Source: CAD feature listing. Evaluate the final solid. Frame: model axes, mm. A direction names the side the tool comes from. Coordinates: 2 decimals unless noted, no trailing zeros. Write each loop counter-clockwise with the first axis right and the second up, starting at its lowest first coordinate (ties: lowest second). Pieces come first, ordered by that corner, then holes. Notation, with made-up numbers: M -38,48.5 L -31,48.5 A26 ccw -31,83.5 Z; hole C 2,52.5 d3. An arc over 180 degrees is marked long. Write item = value, one per line. Start each with the question number.
1. Access query for faces 4 (the face through (4, 84, 3)), 5 (the face through (0, 17, 3)), 6 (the face through (16, 82, 3)). Directions: +Z, -Z, +X, -X, +Y, -Y. A direction counts if a zero-diameter tool reaches every point of the face in a straight line with its end or side. Return the directions, or none.
2. Pull-direction query (Y, two-part tool) for faces 1 (the face through (19.14, 165.1, 3.04)), 2 (the face through (20, 149, 3)), 3 (the face through (3.22, 127.72, 3.04)); classes: pulls with the +Y half, pulls with the -Y half, needs draft (parallel to the pull), parting line crosses it, or undercut.
3. Line query: line 1 along X through (y, z) = (91, 2.1); line 2 along Y through (x, z) = (18.5, 0.3); line 3 along Y through (x, z) = (18.25, 3.75). Output: solid intervals per line, ascending.
4. Section query A-A (z = 3.55). Output: boundary loops of the cut face in (x, y).
5. Section query B-B (y = 95). Output: boundary loops of the cut face in (x, z), then the cut area to 3 significant figures.
Autodesk Inventor part; units mm, degrees
ref_plane "YZ Plane" through (0, 0, 0) normal (1, 0, 0) x (0, 1, 0)
ref_plane "XZ Plane" through (0, 0, 0) normal (0, 1, 0) x (-1, 0, 0)
ref_plane "XY Plane" through (0, 0, 0) normal (0, 0, 1) x (1, 0, 0)
sketch "Skizze1" plane through (0, 0, 0) normal (0, 0, 1) x (1, 0, 0)
  line L0 (0, 0) -> (20, 0)
  line L1 (20, 0) -> (20, 30)
  line L2 (20, 30) -> (0, 30)
  line L3 (0, 30) -> (0, 0)
  line L4 (4, 38) -> (16, 38)
  line L5 (16, 38) -> (16, 128)
  line L6 (16, 128) -> (4, 128)
  line L7 (4, 128) -> (4, 38)
  line L8 (0, 136) -> (20, 136)
  line L9 (20, 136) -> (20, 166)
  line L10 (20, 166) -> (0, 166)
  line L11 (0, 166) -> (0, 136)
  line L12 (0, 136) -> (4, 128)
  line L13 (4, 38) -> (0, 30)
  line L14 (16, 38) -> (20, 30)
  line L15 (20, 136) -> (16, 128)
  point P0 (10, 38)
  point P1 (10, 128)
  dimension "d0" = 20
  dimension "d1" = 30
  dimension "d2" = 20
  dimension "d3" = 30
  dimension "d4" = 10
  dimension "d5" = 90
  dimension "d6" = 8
  dimension "d7" = 8
  dimension "d8" = 10
  dimension "d9" = 12
extrude "Extrusion1" add sketch "Skizze1" along normal blind 6
fillet "Rundung1" radius 3 4 edges at (20, 0, 3) (0, 0, 3) (20, 166, 3) (0, 166, 3)
fillet "Rundung2" radius 30 4 edges at (4, 128, 3) (4, 38, 3) (16, 38, 3) (16, 128, 3)
properties part number "10x5_Probestück"
Results are:
q1.face_4 = +Z, -Z, -X
q1.face_5 = +Z, -Z, -X, +Y, -Y
q1.face_6 = +Z, -Z, +X
q2.face_1 = pulls with the +Y half
q2.face_2 = needs draft
q2.face_3 = undercut
q3.line_1 = 4 to 16
q3.line_2 = 0.4 to 33.09, 132.91 to 165.6
q3.line_3 = 0.27 to 33.68, 132.32 to 165.73
q4.outline = M 0,3 A3 ccw 3,0 L 17,0 A3 ccw 20,3 L 20,30 L 19.17,31.67 A30 cw 16,45.08 L 16,120.92 A30 cw 19.17,134.33 L 20,136 L 20,163 A3 ccw 17,166 L 3,166 A3 ccw 0,163 L 0,136 L 0.83,134.33 A30 cw 4,120.92 L 4,45.08 A30 cw 0.83,31.67 L 0,30 Z
q5.outline = M 4,0 L 16,0 L 16,6 L 4,6 Z
q5.area = 72.0 mm^2
